```python
from build123d import *

# Parameters (mm, degrees)
SKETCH1_R           = 2
BOSS_EXTRUDE1_DEPTH = 1.5
BOSS_EXTRUDE2_DEPTH = 5
SKETCH2_R           = 3.5
SKETCH2_R_2         = 2
BOSS_EXTRUDE3_DEPTH = 1.5
FILLET2_R           = 0.8
FILLET3_R           = 0.5


with BuildPart() as part:
    # Sketch1 → Boss-Extrude1 (new body)
    with BuildSketch(Plane.XY):
        with BuildLine():
            Line((0, -3.5), (20, -3.5))
            ThreePointArc((20, -3.5), (23.5, 0), (20, 3.5))
            Line((20, 3.5), (16.5, 3.5))
            Line((16.5, 3.5), (16.5, 9.5))
            Line((16.5, 9.5), (3.5, 9.5))
            Line((3.5, 9.5), (3.5, 3.5))
            Line((3.5, 3.5), (0, 3.5))
            ThreePointArc((0, 3.5), (-3.5, 0), (0, -3.5))
        make_face()
        with Locations((20, 0)):
            Circle(SKETCH1_R, mode=Mode.SUBTRACT)
        Circle(SKETCH1_R, mode=Mode.SUBTRACT)
    extrude(amount=BOSS_EXTRUDE1_DEPTH)

    # Sketch1_3 → Boss-Extrude2 (add)
    with BuildSketch(Plane.XY):
        with BuildLine():
            ThreePointArc((-3.382776961, 0.898231613), (-2.133798181, 2.774329707), (0, 3.5))
            Line((0, 3.5), (-22, 3.5))
            Line((-22, 3.5), (-22, 0.898231613))
            Line((-22, 0.898231613), (-3.382776961, 0.898231613))
        make_face()
    extrude(amount=BOSS_EXTRUDE2_DEPTH)

    # Sketch2 → Boss-Extrude3 (add)
    # profile 1 of 2: a face of its own
    with BuildSketch(Plane.XY.offset(1.5)):
        with Locations(Location((20, 0, 0), (0, 0, 90))):
            Circle(SKETCH2_R)
        with Locations((20, 0)):
            Circle(SKETCH2_R_2, mode=Mode.SUBTRACT)
    # profile 2 of 2: a face of its own
    with BuildSketch(Plane.XY.offset(1.5)):
        Circle(SKETCH2_R)
        Circle(SKETCH2_R_2, mode=Mode.SUBTRACT)
    extrude(amount=BOSS_EXTRUDE3_DEPTH)

    # Fillet2
    fillet2_edges = [part.edges().sort_by_distance(p)[0] for p in [
        (3.5, 3.5, 0.75),
        (3.5, 9.5, 0.75),
        (16.5, 9.5, 0.75),
        (16.5, 3.5, 0.75),
    ]]
    fillet(fillet2_edges, radius=FILLET2_R)

    # Fillet3
    fillet3_edges = [part.edges().sort_by_distance(p)[0] for p in [
        (-22, 3.5, 2.5),
        (-22, 0.898231613, 2.5),
    ]]
    fillet(fillet3_edges, radius=FILLET3_R)


solid = part.part
```
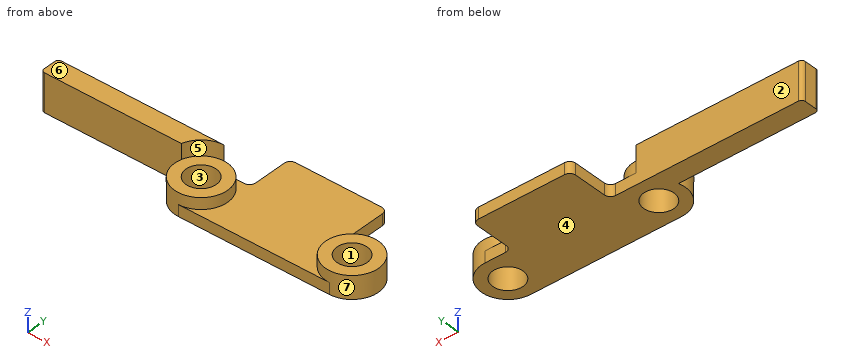
Geometry: final body of the model. Coordinates: model frame, mm. Face numbers are marked on the shaded views. A direction names the side the tool comes from. Coordinates: 2 decimals unless noted, no trailing zeros. Loops run counter-clockwise (first coordinate to the right, second up) from the corner with the lowest first, then second, coordinate; pieces in that order, holes last. Notation, with made-up numbers: M 79.25,-8.75 L 130.25,-8.75 A13 ccw 130.25,-0.75 Z; hole C -36,-13 d11. An arc over 180 degrees is marked long. Put each result on its own line as item: value.
(1) Cut plane B-B on x = 1.5. Return the cut outline in (y, z), then the cut area to 3 significant figures.
Answer sheet:
outline: M -3.5,0 L -1.32,0 L -1.32,3 L -3.16,3 L -3.16,1.5 L -3.5,1.5 Z; M 1.32,0 L 3.5,0 L 3.5,1.5 L 3.16,1.5 L 3.16,3 L 1.32,3 Z
area: 12.0 mm^2
(2) Material intervals for probe 1 along X at (y, z) = (0.75, 1.05); probe 2 along Y at (x, z) = (20, 1.2); probe 3 along X at (y, z) = (-0.25, 0.85), sorted ascending.
Answer sheet:
probe 1: x = -3.42 to -1.85, 1.85 to 18.15, 21.85 to 23.42
probe 2: y = -3.5 to -2, 2 to 3.5
probe 3: x = -3.49 to -1.98, 1.98 to 18.02, 21.98 to 23.49
(3) First-contact query: pin 1 (1.6 mm diameter, centred on x = 18, z = 0.5, fed in from +Y); pin 2 (7.5 mm diameter, centred on x = 0.5, y = -1.5, fed in from +Z); pin 3 (1.5 mm diameter, centred on x = -3, y = 1.5, fed in from -Z); pin 4 (0.8 mm diameter, centred on y = 7, z = 0.5, fed in from +X). Flat tips, straight axial feed; report the tip coordinate or a pass-through.
Answer sheet:
pin 1: stops at y = 3.51
pin 2: stops at z = 3
pin 3: stops at z = 0
pin 4: stops at x = 16.5
(4) Cut plane A-A on z = 1.95. Return the cut outline in (x, y), then the cut area to 3 significant figures.
Answer sheet:
outline: M -22,1.4 A0.5 ccw -21.5,0.9 L -3.38,0.9 A3.5 ccw long 0,3.5 L -21.5,3.5 A0.5 ccw -22,3 Z; C 20,0 d7; hole C 0,0 d4; hole C 20,0 d4
area: 102 mm^2
(5) Cut plane D-D on y = 7.75. Return the cut outline in (x, z), then the cut area to 3 significant figures.
Answer sheet:
outline: M 3.5,0 L 16.5,0 L 16.5,1.5 L 3.5,1.5 Z
area: 19.5 mm^2
(6) Access query for the marked faces 5, 6 and 7. Directions: +Z, -Z, +X, -X, +Y, -Y. A direction counts if a zero-diameter tool reaches every point of the face in a straight line with its end or side. Return the directions, or none.
Answer sheet:
face 5: +Z, +X, -Y
face 6: +Z, +X, -X, +Y, -Y
face 7: +Z
(7) Cut plane C-C on x = 8. Return the cut outline in (y, z).
Answer sheet:
outline: M -3.5,0 L 9.5,0 L 9.5,1.5 L -3.5,1.5 Z
(8) Draft query along Y for the marked faces 1, 2, 3 and 4. Return one class per face: pulls with the +Y half, pulls with the -Y half, needs draft (parallel to the pull), parting line crosses it, or undercut.
Answer sheet:
face 1: undercut
face 2: pulls with the +Y half
face 3: undercut
face 4: needs draft
